Autodesk Inventor part; units mm, degrees
ref_plane "Work Plane1" through (0, 3, 0) normal (0, 0.8036, 0.5952) x (1, 0, 0)
ref_plane "Work Plane2" through (20, 0, -21) normal (-1, 0, 0) x (0, 0, 1)
ref_plane "YZ Plane" through (0, 0, 0) normal (1, 0, 0) x (0, 1, 0)
sketch "Sketch1" plane through (0, 0, 0) normal (0, 1, 0) x (-1, 0, 0)
  line L0 (0, 0) -> (-40, 0)
  line L1 (-40, 0) -> (-40, -21)
  line L2 (-40, -21) -> (0, -21)
  line L3 (0, -21) -> (0, 0)
  circle A0 centre (-7.5, -10) radius 2.65
  circle A1 centre (-32.5, -10) radius 2.65
  line L4 (-7.5, -10) -> (-32.5, -10) construction
  line L5 (0, -21) -> (-40, -21)
  line L6 (-40, -21) -> (-40, -18)
  line L7 (-40, -18) -> (0, -18)
  line L8 (0, -18) -> (0, -21)
  line L9 (-40, -21) -> (-39, -21)
  line L10 (-39, -21) -> (-39, 0)
  line L11 (-39, 0) -> (-40, 0)
  line L12 (-40, 0) -> (-40, -21)
  line L13 (0, 0) -> (-1, 0)
  line L14 (-1, 0) -> (-1, -21)
  line L15 (-1, -21) -> (0, -21)
  line L16 (0, -21) -> (0, 0)
  line L17 (-32.5, -10) -> (-40, -10) construction
  line L18 (-7.5, -10) -> (0, -10) construction
  point P0 (-1, -18)
  point P1 (-39, -18)
  dimension "d0" = 40
  dimension "d1" = 21
  dimension "d3" = 5.3
  dimension "d4" = 3
  dimension "d9" = 1
  dimension "d10" = 1
  dimension "d23" = 11
  dimension "d24" = 25
extrude "Extrusion1" add sketch "Sketch1" along normal blind 3
extrude "Extrusion2" add sketch "Sketch1" along normal blind 16.3333 contours L3 L2 L14 L7 | L14 L2 L10 L7 | L10 L2 L1 L7
ref_plane "Work Plane1" through (0, 3, 0) normal (0, 0.8036, 0.5952) x (1, 0, 0)
extrude "Extrusion3" add sketch "Sketch1" along normal up to surface contours L3 L7 L14 L0 | L10 L7 L1 L0 surface through (0, 3, 0) normal (0, 0.8036, 0.5952)
sketch "Sketch3" plane through (1, 3, -18) normal (0, 0, 1) x (1, 0, 0)
  line L0 (0, 13.3333) -> (0, 0)
  line L1 (0, 13.3333) -> (0, 0)
  line L2 (38, 0) -> (0, 0)
  line L3 (38, 0) -> (38, 13.3333)
  line L4 (0, 13.3333) -> (38, 13.3333)
  line L5 (0, 6.6667) -> (7.5, 6.6667) construction
  line L6 (7.5, 6.6667) -> (30.5, 6.6667) construction
  line L7 (30.5, 6.6667) -> (38, 6.6667) construction
  circle A0 centre (7.5, 6.6667) radius 2.65
  circle A1 centre (30.5, 6.6667) radius 2.65
  point P0 (-1, -3)
  dimension "d13" = 7.5
  dimension "d14" = 5.3
extrude "Extrusion4" cut sketch "Sketch3" against normal through all contours A0 | A1
ref_plane "Work Plane2" through (20, 0, -21) normal (-1, 0, 0) x (0, 0, 1)
sketch "Sketch5" plane through (0, 0, 0) normal (0, -1, 0) x (1, 0, 0)
  line L0 (0, -5.625) -> (40, -5.625)
  line L1 (40, -5.625) -> (40, -14.375)
  line L2 (40, -14.375) -> (0, -14.375)
  line L3 (0, -14.375) -> (0, -5.625)
  line L4 (0, -21) -> (0, 0)
  line L5 (40, 0) -> (40, -21)
  line L6 (0, -10) -> (40, -10) construction
  circle A0 centre (7.5, -10) radius 2.65
  circle A1 centre (32.5, -10) radius 2.65
  dimension "d17" = 8.75
extrude "Extrusion5" add sketch "Sketch5" along normal blind 1.35
chamfer "Chamfer1" distance 1.35 angle 45 2 edges at (20, -1.35, -5.625) (20, -1.35, -14.375)
fillet "Fillet1" radius 2 5 edges at (1, 3, -9) (1, 9.6667, -18) (20, 3, -18) (39, 9.6667, -18) (39, 3, -9)
sketch "Sketch6" plane through (3, 5, -18) normal (0, 0, 1) x (1, 0, 0)
  circle A0 centre (28.5, 4.6667) radius 2.65
  circle A1 centre (5.5, 4.6667) radius 2.65
  circle A2 centre (5.5, 4.6667) radius 4.25
  circle A3 centre (28.5, 4.6667) radius 4.25
  point P0 (-3, -5)
  dimension "d26" = 8.5
  dimension "d27" = 8.5
extrude "Extrusion6" add sketch "Sketch6" along normal blind 5
sketch "Sketch7" plane through (0, 3, 0) normal (0, 1, 0) x (1, 0, 0)
  circle A0 centre (7.5, 10) radius 2.65
  circle A1 centre (32.5, 10) radius 2.65
  circle A2 centre (7.5, 10) radius 4.25
  circle A3 centre (32.5, 10) radius 4.25
  point P0 (0, 0)
  dimension "d30" = 8.5
  dimension "d31" = 8.5
extrude "Extrusion7" add sketch "Sketch7" along normal blind 5
properties part number "Soporte Cajas" material "Rubber, Silicone"
Geometry check sheet. Reference: the model listing, model coordinates, mm. A direction names the side the tool comes from. Coordinates: 2 decimals unless noted, no trailing zeros. Order: outer loops, then holes, each group sorted by start corner. A loop starts at its lowest first (then second) coordinate and runs counter-clockwise, first axis right, second up. Notation, with made-up numbers: M 51,-5.75 L 89,-5.75 A20 cw 89,29.25 Z; hole C 23,16.5 d3. An arc over 180 degrees is marked long. One line per question, with ' | ' between items. Start each with the question number.
Item 1: Draft check along Z on faces 6 (the cylindrical face through (6.947, 5.465, -5.786)), 7 (the flat face through (20, 16.333, -19)), 8 (the cylindrical face through (1.6, 10.75, -17.43)). Enter one of: pulls with the +Z half, pulls with the -Z half, needs draft (parallel to the pull), parting line crosses it, or undercut.
Item 2: Cross-section at B-B on x = 8.5. State how many separate pieces and enclosed holes the cut face has, then the cut area to 3 significant figures.
Item 3: Cross-section at C-C on z = -8.5. Enter the section's corners in (x, y).
Item 4: Set-up check for faces 1 (the cylindrical face through (1.57, 3.6, -7.89)), 2 (the cylindrical face through (20.24, 3.57, -17.4)), 3 (the flat face through (20, 0, -18)), 4 (the flat face through (20, 0, -3)), 5 (the flat face through (0.396, 9.697, -9.042)): record each of +Z, -Z, +X, -X, +Y, -Y from which the full face is reachable in a straight line by a thin tool's end or side.
Item 5: Material ranges on L1, parallel to X at y = 2.2, z = -10; L2, parallel to Y at x = 8.5, z = -15.35; L3, parallel to Z at x = 7.5, y = 2, recorded low to high. Write a range as [from, to].
Item 6: Cross-section at D-D on y = 2. Enter the section's corners in (x, z), then the cut area to 3 significant figures.
Item 7: Gauge pin test, flat ends, axial feed: pin 1 (4 mm diameter, centred on x = 9, z = -10.5, fed in from +Y); pin 2 (4 mm diameter, centred on x = 31.5, y = 9.67, fed in from -Z); pin 3 (9 mm diameter, centred on x = 32.5, y = 8, fed in from +Z). Record the tip position at first contact, or that the pin passes through.
Findings:
1) face 6: undercut | face 7: needs draft | face 8: pulls with the +Z half
2) separate pieces: 3 | enclosed holes: 1 | area: 108 mm²
3) outline: M 0,-1.35 L 5.32,-1.35 L 5.32,8 L 3.52,8 L 3.52,3 L 3,3 A2 cw 1,5 L 1,9.3 L 0,9.3 Z; M 9.68,-1.35 L 30.32,-1.35 L 30.32,8 L 28.52,8 L 28.52,3 L 11.48,3 L 11.48,8 L 9.68,8 Z; M 34.68,-1.35 L 40,-1.35 L 40,9.3 L 39,9.3 L 39,5 A2 cw 37,3 L 36.48,3 L 36.48,8 L 34.68,8 Z
4) face 1: +Z, +Y | face 2: none | face 3: -Z, +X, -X, -Y | face 4: +Z, +X, -X, -Y | face 5: +Z, -X, +Y
5) L1: x = [0, 4.85], [10.15, 29.85], [35.15, 40] | L2: y = [0, 3], [5.42, 7.02], [12.32, 13.92] | L3: z = [-21, -12.65], [-7.35, 0]
6) outline: M 0,-21 L 40,-21 L 40,0 L 0,0 Z; hole C 7.5,-10 d5.3; hole C 32.5,-10 d5.3 | area: 796 mm²
7) pin 1: stops at y = 8 | pin 2: stops at z = -14.25 | pin 3: stops at z = -5.75
